```python
from build123d import *

# Parameters (mm, degrees)
SKETCH_1_R          = 3
EXTRUDE_1_DEPTH     = 1.5
CUT_EXTRUDE_1_DEPTH = 22
FILLET_1_R          = 2


with BuildPart() as part:
    # 草图1 → 凸台-拉伸1 (new, symmetric)
    with BuildSketch(Plane.XY):
        with BuildLine():
            Line((-1.233702436, 4.84540796), (14.292269552, 8.798517714))
            Line((14.292269552, 8.798517714), (27.541816671, 8.302545362))
            Line((27.541816671, 8.302545362), (50.285691672, 7.168894271))
            Line((50.285691672, 7.168894271), (48.971743891, -1.387225717))
            Line((48.971743891, -1.387225717), (38.114277377, -2.724152564))
            Line((38.114277377, -2.724152564), (18.384478153, -4.790312237))
            Line((18.384478153, -4.790312237), (3.124153733, -7.364758207))
            Line((3.124153733, -7.364758207), (-2.372822781, -4.401103504))
            ThreePointArc((-2.372822781, -4.401103504), (-4.962484216, 0.611351292), (-1.233702436, 4.84540796))
        make_face()
        Circle(SKETCH_1_R, mode=Mode.SUBTRACT)
    extrude(amount=EXTRUDE_1_DEPTH, both=True)

    # 草图2 → 切除-拉伸1 (cut)
    with BuildSketch(Plane.XY.offset(1.5)):
        with BuildLine():
            ThreePointArc((6, -2.05), (26.381158068, -1.352479883), (46.666940766, 0.736816365))
            ThreePointArc((46.666940766, 0.736816365), (47.563889378, 1.920236488), (46.380469254, 2.8171851))
            ThreePointArc((46.380469254, 2.8171851), (26.237586384, 0.742606553), (6, 0.05))
            ThreePointArc((6, 0.05), (4.95, -1), (6, -2.05))
        make_face()
    extrude(amount=-CUT_EXTRUDE_1_DEPTH, mode=Mode.SUBTRACT)

    # 圆角1
    fillet_1_edges = [part.edges().sort_by_distance(p)[0] for p in [
        (14.292269552, 8.798517714, 0),
        (27.541816671, 8.302545362, 0),
        (50.285691672, 7.168894271, 0),
        (48.971743891, -1.387225717, 0),
        (38.114277377, -2.724152564, 0),
        (18.384478153, -4.790312237, 0),
        (3.124153733, -7.364758207, 0),
    ]]
    fillet(fillet_1_edges, radius=FILLET_1_R)


solid = part.part
```
The listing builds one solid part. Answer for the finished solid, in the listing's coordinates (mm). A direction names the side the tool comes from. Coordinates: 2 decimals unless noted, no trailing zeros. Loops run counter-clockwise (first coordinate to the right, second up) from the corner with the lowest first, then second, coordinate; pieces in that order, holes last. Notation, with made-up numbers: M -20,1 L -11,1 A27 ccw -11,25 Z; hole C 23,59.5 d9. An arc over 180 degrees is marked long. Answer as CSV lines item,"result". Start each with the question number.
(1) The mould has two halves that part along Y. Classify faces 3 (the cylindrical face through (26.52, 0.762, 0.021)), 4 (the flat face through (49.58, 2.58, 0.02)), 5 (the flat face through (37.66, 7.8, 0.02)): pulls with the +Y half, pulls with the -Y half, needs draft (parallel to the pull), parting line crosses it, or undercut.
(2) Find the intervals of material crossed by L1, parallel to Y at x = 0, z = -0.3; L2, parallel to Y at x = 21.5, z = -0.45; L3, parallel to X at y = 3.5, z = -1.15, in increasing order. Write a range as [from, to].
(3) The part is cut by section D-D (x = 5.5). Give the vertices of the cut face in (y, z), and give its area (3 significant figures).
(4) The part is cut by section B-B (x = 21). Give the vertices of the cut face in (y, z).
(5) For faces 1 (the cylindrical face through (47.567, 1.897, 0.021)), 2 (the flat face through (20.97, 8.55, 0.02)), determine the directions among +Z, -Z, +X, -X, +Y, -Y from which every point of the face is accessible in a straight line to the end or side of a thin tool.
(6) The part is cut by section A-A (z = -0.05). Give the vertices of the cut face in (x, y), and give its area (3 significant figures).
(7) The part is cut by section C-C (y = -1). Give the vertices of the cut face in (x, z).
Determined:
1,face 3,"undercut"
1,face 4,"pulls with the -Y half"
1,face 5,"pulls with the +Y half"
2,L1,"[-5.68, -3], [3, 5.16]"
2,L2,"[-4.46, -1.65], [0.46, 8.53]"
2,L3,"[-3.57, 49.72]"
3,outline,"M -6.96,-1.5 L -1.92,-1.5 L -1.92,1.5 L -6.96,1.5 Z; M -0.08,-1.5 L 6.56,-1.5 L 6.56,1.5 L -0.08,1.5 Z"
3,area,"35.0 mm2"
4,outline,"M -4.52,-1.5 L -1.67,-1.5 L -1.67,1.5 L -4.52,1.5 Z; M 0.43,-1.5 L 8.55,-1.5 L 8.55,1.5 L 0.43,1.5 Z"
5,face 1,"+Z, -Z"
5,face 2,"+Z, -Z, +X, +Y"
6,outline,"M -2.37,-4.4 L 2.52,-7.04 A2 ccw 3.8,-7.25 L 18.38,-4.79 L 38.11,-2.72 L 47.47,-1.57 A2 ccw 49.2,0.11 L 49.95,4.98 A2 ccw 48.07,7.28 L 27.54,8.3 L 14.58,8.79 A2 ccw 14.01,8.73 L -1.23,4.85 A5 ccw Z; hole C 0,0 d6; hole M 6,-2.05 A298.11 ccw 46.67,0.74 A1.05 ccw 46.38,2.82 A296.01 cw 6,0.05 A1.05 ccw Z"
6,area,"516 mm2"
7,outline,"M -4.9,-1.5 L -2.83,-1.5 L -2.83,1.5 L -4.9,1.5 Z; M 2.83,-1.5 L 4.95,-1.5 L 4.95,1.5 L 2.83,1.5 Z; M 31,-1.5 L 48.64,-1.5 L 48.64,1.5 L 31,1.5 Z"
